from build123d import *

# Parameters (mm, degrees)
F1_DEPTH = 15
F2_R     = 5
F3_R     = 5
F5_D     = 3
F7_D     = 3


with BuildPart() as f1:
    # F0 (on Right) → F1 (new body)
    with BuildSketch(Plane.YZ):
        Polygon((-2, -38), (0, -38), (0, 0), (38, 0), (38, 2), (-2, 2), align=None)
    extrude(amount=F1_DEPTH)

    # F2
    f2_edges = [f1.edges().sort_by_distance(p)[0] for p in [
        (7.5, -2, 2),
    ]]
    fillet(f2_edges, radius=F2_R)

    # F3
    f3_edges = [f1.edges().sort_by_distance(p)[0] for p in [
        (7.5, 0, 0),
    ]]
    fillet(f3_edges, radius=F3_R)

    # F5 (through all)
    with Locations(Plane.XY.offset(2)):
        with Locations((7.5, 24.5), (7.5, 16.5)):
            Hole(F5_D / 2)

    # F7 (through all)
    with Locations(Plane.XZ.offset(2)):
        with Locations((7.5, -8), (7.5, -28)):
            Hole(F7_D / 2)


solid = f1.part
Geometry: final body of the model. Coordinates: model frame, mm. A direction names the side the tool comes from. Round coordinates to 2 decimals unless told otherwise and drop trailing zeros. Order: outer loops, then holes, each group sorted by start corner. A loop starts at its lowest first (then second) coordinate and runs counter-clockwise, first axis right, second up. Notation, with made-up numbers: (2, 79) -> (13, 79) arc R22 cw to (13, 105) -> close; hole circle Ø6 at (-21.5, 54). An arc over 180 degrees is marked (long way). Put each result on its own line as item: value. Start each with the question number.
Q1. Reachability of faces 5 (the flat face through (7, -2, -20)), 6 (the flat face through (7, 21, 0)) from +Z, -Z, +X, -X, +Y, -Y: full face, straight path, thin tool, end or side. Return the list, or none.
Q2. Section A-A on x = 7.5. Return the cut outline in (y, z), and give its area (3 significant figures).
Q3. Section B-B on z = -28. Return the cut outline in (x, y).
Q4. Section D-D on x = 10. Return the cut outline in (y, z).
Q5. Pull-direction query (Z, two-part tool) for faces 1 (the cylindrical face through (7.695, -0.986, -26.513)), 2 (the cylindrical face through (8.7, -1, -8.9)), 3 (the flat face through (7, -1, -38)), 4 (the flat face through (7, 21, 2)); classes: +Z half, -Z half, draft (parallel to the pull), parting line (faces both ways), or undercut.
Q6. Line query: probe 1 along Z at (x, y) = (7.5, -1); probe 2 along Y at (x, z) = (7.5, 0.65); probe 3 along Z at (x, y) = (7.5, -1.35). Output: solid intervals per line, ascending.
Q7. First-contact query: pin 1 (4 mm diameter, centred on y = 3.5, z = -8, fed in from -X); pin 2 (5 mm diameter, centred on x = 7.5, z = -28, fed in from +Y); pin 3 (4 mm diameter, centred on x = 7.5, y = 24.5, fed in from -Z); pin 4 (1 mm diameter, centred on x = 11, z = -4.5, fed in from +Y). Flat tips, straight axial feed; report the tip coordinate or a pass-through.
Q8. Section C-C on y = 24.5. Return the cut outline in (x, z), and give its area (3 significant figures).
Ans:
1. face 5: +Z, -Z, +X, -X, -Y
1. face 6: -Z, +X, -X, +Y
2. outline: (-2, -38) -> (0, -38) -> (0, -29.5) -> (-2, -29.5) -> close; (-2, -26.5) -> (0, -26.5) -> (0, -9.5) -> (-2, -9.5) -> close; (-2, -6.5) -> (0, -6.5) -> (0, -5) arc R5 cw to (5, 0) -> (15, 0) -> (15, 2) -> (3, 2) arc R5 ccw to (-2, -3) -> close; (18, 0) -> (23, 0) -> (23, 2) -> (18, 2) -> close; (26, 0) -> (38, 0) -> (38, 2) -> (26, 2) -> close
2. area: 132 mm2
3. outline: (0, -2) -> (6, -2) -> (6, 0) -> (0, 0) -> close; (9, -2) -> (15, -2) -> (15, 0) -> (9, 0) -> close
4. outline: (-2, -38) -> (0, -38) -> (0, -5) arc R5 cw to (5, 0) -> (38, 0) -> (38, 2) -> (3, 2) arc R5 ccw to (-2, -3) -> close
5. face 1: undercut
5. face 2: undercut
5. face 3: -Z half
5. face 4: +Z half
6. probe 1: z = -38 to -29.5, -26.5 to -9.5, -6.5 to 0
6. probe 2: y = -0.42 to 15, 18 to 23, 26 to 38
6. probe 3: z = -38 to -29.5, -26.5 to -9.5, -6.5 to -0.53
7. pin 1: passes through
7. pin 2: stops at y = 0
7. pin 3: stops at z = 0
7. pin 4: stops at y = 0.1
8. outline: (0, 0) -> (6, 0) -> (6, 2) -> (0, 2) -> close; (9, 0) -> (15, 0) -> (15, 2) -> (9, 2) -> close
8. area: 24.0 mm2
